The listing builds one solid part. Answer for the finished solid, in the listing's coordinates (mm). A direction names the side the tool comes from. Give positions to 0.01 mm unless a question says otherwise; leave off trailing zeros. Order: outer loops, then holes, each group sorted by start corner. A loop starts at its lowest first (then second) coordinate and runs counter-clockwise, first axis right, second up. Notation, with made-up numbers: (60.5, 61) - (64.5, 61) arc R32 ccw to (64.5, 96) - close; hole circle Ø8 at (88.25, 24). An arc over 180 degrees is marked (long way). Write each question's results on one line, items separated by ' | '. Start each with the question number.
1. Determine the mould class of faces 1 (the face through (-13, 30, 0)), 2 (the face through (92.2, 27.1, -89.24)), 3 (the face through (98.12, 31, -64)), 4 (the face through (58, 52, -33)) for opening direction Z: released by +Z, released by -Z, zero draft, split by the parting line, or undercut.
2. Section A-A (z = -94) is taken. Give the vertices of the cut face in (x, y), and give its area (4 significant figures).
3. Section C-C (z = -22.5) is taken. Give the vertices of the cut face in (x, y), and give its area (3 significant figures).
4. Find the intervals of material crossed by L1, parallel to X at y = 49.5, z = -27; L2, parallel to X at y = 11, z = -124; L3, parallel to Y at x = -123, z = -109.25, in increasing order.
5. Section B-B (z = -53) is taken. Give the vertices of the cut face in (x, y).
6. Flat-ended cylindrical pins translate along their axes: pin 1 (5 mm diameter, centred on x = 92.12, z = -5, fed in from -Y); pin 2 (3 mm diameter, centred on x = -123.62, z = -5, fed in from +Y); pin 3 (2 mm diameter, centred on x = 59.5, y = 53.5, fed in from -Z); pin 4 (10 mm diameter, centred on x = 56, y = 15, fed in from -Z). Find the tip coordinate at first contact, or state that the pin passes through.
7. Which of the six approach directions +Z, -Z, +X, -X, +Y, -Y give full straight-line access (tool end or side, diameter ignored) to faces 5 (the face through (-82.38, 9, -5)), 6 (the face through (58, 49, -19)), 7 (the face through (-120.12, 30, -70)), 8 (the face through (-124, 30, -129))?
from build123d import *

# Parameters (mm, degrees)
SKETCH1_W                      = 129
SKETCH1_H                      = 55.5
BOSS_EXTRUDE1_DEPTH            = 98.12
SKETCH18_W                     = 129
SKETCH18_H                     = 55.5
BOSS_EXTRUDE9_DEPTH            = 29
SKETCH33_W                     = 156
SKETCH33_H                     = 12.5
CUT_EXTRUDE8_DEPTH             = 20.5
SKETCH40_W                     = 206.24
SKETCH40_H                     = 49.5
CUT_EXTRUDE9_DEPTH             = 119
CUT_EXTRUDE18_REACH            = 191.422
SKETCH62_W                     = 8.5
SKETCH62_H                     = 3.5
M4_CLEARANCE_HOLE2_D           = 4.5
F_2_0_221_DIAMETER_HOLE1_D     = 2.50000008
F_2_0_221_DIAMETER_HOLE1_DEPTH = 20
F_2_0_221_DIAMETER_HOLE1_TIP   = 0.751075798
SKETCH70_W                     = 32
SKETCH70_H                     = 6.5
BOSS_EXTRUDE10_DEPTH           = 23
SKETCH71_W                     = 26
SKETCH71_H                     = 3.5
CUT_EXTRUDE19_DEPTH            = 30
SKETCH73_W                     = 225.24
SKETCH73_H                     = 6
CUT_EXTRUDE20_DEPTH            = 190.422132815
F_3_7_3_7_DIAMETER_HOLE1_D     = 3.7
F_3_7_3_7_DIAMETER_HOLE1_DEPTH = 12
F_3_7_3_7_DIAMETER_HOLE1_TIP   = 1.111592145
F_3_7_3_7_DIAMETER_HOLE2_D     = 3.7
F_3_7_3_7_DIAMETER_HOLE2_DEPTH = 12
F_3_7_3_7_DIAMETER_HOLE2_TIP   = 1.111592145
M4_CLEARANCE_HOLE3_D           = 4.5
M4_CLEARANCE_HOLE3_DEPTH       = 12
M4_CLEARANCE_HOLE3_TIP         = 1.351936393
F_3_CLEARANCE_HOLE1_D          = 2.794
F_3_CLEARANCE_HOLE1_DEPTH      = 7
F_12_0MM_DOWEL_HOLE1_D         = 12
F_12_0MM_DOWEL_HOLE1_DEPTH     = 12


with BuildPart() as part:
    # Sketch1 → Boss-Extrude1 (new, symmetric)
    with BuildSketch(Plane(origin=(0, 0, 0), x_dir=(0, 0, -1), z_dir=(1, 0, 0))):
        with Locations((64.5, 27.75)):
            Rectangle(SKETCH1_W, SKETCH1_H)
    extrude(amount=BOSS_EXTRUDE1_DEPTH, both=True)

    # Sketch18 → Boss-Extrude9 (add)
    with BuildSketch(Plane.ZY.offset(98.12)):
        with Locations((-64.5, 27.75)):
            Rectangle(SKETCH18_W, SKETCH18_H)
    extrude(amount=BOSS_EXTRUDE9_DEPTH)

    # Sketch33 → Cut-Extrude8 (cut)
    with BuildSketch(Plane.XY):
        with Locations((-4.38, 6.25)):
            Rectangle(SKETCH33_W, SKETCH33_H)
    extrude(amount=-CUT_EXTRUDE8_DEPTH, mode=Mode.SUBTRACT)

    # Sketch40 → Cut-Extrude9 (cut)
    with BuildSketch(Plane(origin=(0, 0, -129), x_dir=(-1, 0, 0), z_dir=(0, 0, -1))):
        with Locations((17, 30.75)):
            Rectangle(SKETCH40_W, SKETCH40_H)
    extrude(amount=-CUT_EXTRUDE9_DEPTH, mode=Mode.SUBTRACT)

    # Sketch62 → Cut-Extrude18 (cut, up to next)
    with BuildSketch(Plane.XY, mode=Mode.PRIVATE) as cut_extrude18_sk1:
        with Locations((-105.87, 18.25)):
            Rectangle(SKETCH62_W, SKETCH62_H)
    cut_extrude18_tool1 = extrude(cut_extrude18_sk1.sketch, amount=-CUT_EXTRUDE18_REACH, mode=Mode.PRIVATE) & part.part
    add(cut_extrude18_tool1.solids().sort_by_distance((-105.87, 18.25, 0))[0], mode=Mode.SUBTRACT)

    # M4 Clearance Hole2 (through all)
    with Locations(Plane.XY):
        with Locations((-34.375, 18.75), (25.625, 18.75)):
            Hole(M4_CLEARANCE_HOLE2_D / 2)

    # #2 (0.221) Diameter Hole1
    with Locations(Plane(origin=(0, 0, -129), x_dir=(-1, 0, 0), z_dir=(0, 0, -1))):
        with Locations((-91.573125, 38.6875), (-91.573125, 22.8125)):
            Hole(F_2_0_221_DIAMETER_HOLE1_D / 2, depth=F_2_0_221_DIAMETER_HOLE1_DEPTH)
            with Locations((0, 0, -(F_2_0_221_DIAMETER_HOLE1_DEPTH + F_2_0_221_DIAMETER_HOLE1_TIP / 2))):  # 118° drill point
                Cone(0, F_2_0_221_DIAMETER_HOLE1_D / 2, F_2_0_221_DIAMETER_HOLE1_TIP, mode=Mode.SUBTRACT)

    # Sketch70 → Boss-Extrude10 (add)
    with BuildSketch(Plane(origin=(0, 0, -10), x_dir=(-1, 0, 0), z_dir=(0, 0, -1))):
        with Locations((-57.63, 52.25)):
            Rectangle(SKETCH70_W, SKETCH70_H)
    extrude(amount=BOSS_EXTRUDE10_DEPTH)

    # Sketch71 → Cut-Extrude19 (cut)
    with BuildSketch(Plane.XY):
        with Locations((57.63, 53.75)):
            Rectangle(SKETCH71_W, SKETCH71_H)
    extrude(amount=-CUT_EXTRUDE19_DEPTH, mode=Mode.SUBTRACT)

    # Sketch73 → Cut-Extrude20 (cut, through all)
    with BuildSketch(Plane(origin=(0, 0, -129), x_dir=(-1, 0, 0), z_dir=(0, 0, -1))):
        with Locations((14.5, 3)):
            Rectangle(SKETCH73_W, SKETCH73_H)
    extrude(amount=-CUT_EXTRUDE20_DEPTH, mode=Mode.SUBTRACT)

    # Ø3.7 (3.7) Diameter Hole1
    with Locations(Plane(origin=(0, 55.5, 0), x_dir=(1, 0, 0), z_dir=(0, 1, 0))):
        with Locations((92.12, 124), (92.12, 5), (-123.62, 124), (-123.62, 5), (23.14, 5), (-21.86, 5)):
            Hole(F_3_7_3_7_DIAMETER_HOLE1_D / 2, depth=F_3_7_3_7_DIAMETER_HOLE1_DEPTH)
            with Locations((0, 0, -(F_3_7_3_7_DIAMETER_HOLE1_DEPTH + F_3_7_3_7_DIAMETER_HOLE1_TIP / 2))):  # 118° drill point
                Cone(0, F_3_7_3_7_DIAMETER_HOLE1_D / 2, F_3_7_3_7_DIAMETER_HOLE1_TIP, mode=Mode.SUBTRACT)

    # Ø3.7 (3.7) Diameter Hole2
    with Locations(Plane(origin=(0, 6, 0), x_dir=(-1, 0, 0), z_dir=(0, -1, 0))):
        with Locations((-92.12, 124), (-92.12, 5), (123.62, 5), (123.62, 124)):
            Hole(F_3_7_3_7_DIAMETER_HOLE2_D / 2, depth=F_3_7_3_7_DIAMETER_HOLE2_DEPTH)
            with Locations((0, 0, -(F_3_7_3_7_DIAMETER_HOLE2_DEPTH + F_3_7_3_7_DIAMETER_HOLE2_TIP / 2))):  # 118° drill point
                Cone(0, F_3_7_3_7_DIAMETER_HOLE2_D / 2, F_3_7_3_7_DIAMETER_HOLE2_TIP, mode=Mode.SUBTRACT)

    # M4 Clearance Hole3
    with Locations(Plane(origin=(0, 52, 0), x_dir=(1, 0, 0), z_dir=(0, 1, 0))):
        with Locations((57.63, 22.5)):
            Hole(M4_CLEARANCE_HOLE3_D / 2, depth=M4_CLEARANCE_HOLE3_DEPTH)
            with Locations((0, 0, -(M4_CLEARANCE_HOLE3_DEPTH + M4_CLEARANCE_HOLE3_TIP / 2))):  # 118° drill point
                Cone(0, M4_CLEARANCE_HOLE3_D / 2, M4_CLEARANCE_HOLE3_TIP, mode=Mode.SUBTRACT)

    # #3 Clearance Hole1
    with Locations(Plane.ZY.offset(127.12)):
        with Locations((-109.25, 41.5), (-109.25, 20)):
            Hole(F_3_CLEARANCE_HOLE1_D / 2, depth=F_3_CLEARANCE_HOLE1_DEPTH)

    # Ø12.0mm Dowel Hole1
    with Locations(Plane.ZY.offset(-86.12)):
        with Locations((-94, 30.75)):
            Hole(F_12_0MM_DOWEL_HOLE1_D / 2, depth=F_12_0MM_DOWEL_HOLE1_DEPTH)


solid = part.part
Reported:
1) face 1: released by +Z | face 2: undercut | face 3: zero draft | face 4: released by -Z
2) outline: (-127.12, 6) - (-120.12, 6) - (-120.12, 55.5) - (-127.12, 55.5) - close; (86.12, 6) - (98.12, 6) - (98.12, 24.75) - (86.12, 24.75) - close; (86.12, 36.75) - (98.12, 36.75) - (98.12, 55.5) - (86.12, 55.5) - close | area: 796.5 mm²
3) outline: (-127.12, 6) - (-120.12, 6) - (-120.12, 55.5) - (-127.12, 55.5) - close; (41.63, 49) - (55.38, 49) - (55.38, 52) - (44.63, 52) - (44.63, 55.5) - (41.63, 55.5) - close; (59.88, 49) - (73.63, 49) - (73.63, 55.5) - (70.63, 55.5) - (70.63, 52) - (59.88, 52) - close; (86.12, 6) - (98.12, 6) - (98.12, 55.5) - (86.12, 55.5) - close | area: 1,040 mm²
4) L1: -127.12 to -120.12, 41.63 to 73.63, 86.12 to 98.12 | L2: -127.12 to -125.47, -121.77 to -120.12, 86.12 to 90.27, 93.97 to 98.12 | L3: 6 to 18.6, 21.4 to 40.1, 42.9 to 55.5
5) outline: (-127.12, 6) - (-120.12, 6) - (-120.12, 55.5) - (-127.12, 55.5) - close; (86.12, 6) - (98.12, 6) - (98.12, 55.5) - (86.12, 55.5) - close
6) pin 1: y = 6 | pin 2: y = 43.29 | pin 3: z = -33 | pin 4: z = -10
7) face 5: +Z, -Z, -Y | face 6: -Z, -Y | face 7: -Z, +Y, -Y | face 8: -Z, +X, -X, +Y, -Y
